Autodesk Inventor part; units mm, degrees
ref_plane "YZ Plane" through (0, 0, 0) normal (1, 0, 0) x (0, 1, 0)
ref_plane "XZ Plane" through (0, 0, 0) normal (0, 1, 0) x (-1, 0, 0)
ref_plane "XY Plane" through (0, 0, 0) normal (0, 0, 1) x (1, 0, 0)
sketch "Sketch1" plane through (0, 0, 0) normal (0, 1, 0) x (-1, 0, 0)
  line L0 (0, 22.5) -> (12, 22.5)
  line L1 (12, 22.5) -> (12, -22.5)
  line L2 (12, -22.5) -> (0, -22.5)
  arc A0 (0, -6.15) -> (0, 6.15) centre (0, 0) ccw
  line L3 (0, 22.5) -> (0, 6.15)
  line L4 (0, -6.15) -> (0, -22.5)
  point P0 (12, 0)
  dimension "d0" = 12
  dimension "d1" = 45
  dimension "d2" = 6.15
extrude "Extrusion1" add sketch "Sketch1" along normal blind 8
sketch "Sketch2" plane through (0, 8, 0) normal (0, 1, 0) x (1, 0, 0)
  line L0 (0, -22.5) -> (0, -6.15)
  arc A0 (0, 7.65) -> (0, -7.65) centre (0, 0) ccw
  line L1 (0, -7.65) -> (0, 7.65)
  dimension "d5" = 7.65
extrude "Extrusion2" cut sketch "Sketch2" against normal blind 3
sketch "Sketch3" plane through (0, 0, 22.5) normal (1, 0, 0) x (0, 0, -1)
  circle A0 centre (6.5, 4) radius 1.6
  circle A1 centre (38.5, 4) radius 1.6
  line L0 (16.35, 0) -> (0, 0)
  point P0 (22.5, 0)
  dimension "d8" = 3.2
  dimension "d9" = 32
  dimension "d10" = 4
  dimension "d11" = 16
extrude "Extrusion3" cut sketch "Sketch3" against normal up to next
sketch "Sketch4" plane through (0, 8, 0) normal (0, 1, 0) x (1, 0, 0)
  line L0 (-12, 22.5) -> (0, 22.5)
  line L1 (0, 22.5) -> (0, 14.5)
  line L2 (0, 14.5) -> (-12, 14.5)
  line L3 (-12, 14.5) -> (-12, 22.5)
  point P0 (0, 0)
  dimension "d14" = 8
extrude "Extrusion4" add sketch "Sketch4" along normal blind 20
sketch "Sketch5" plane through (0, 28, 0) normal (0, 1, 0) x (1, 0, 0)
  line L0 (10.0416, 49.5) -> (-12, 49.5)
  line L1 (-12, 49.5) -> (-12, 14.5)
  arc A0 (-2, 14.5) -> (15, 31.5) centre (-2, 31.5) ccw
  line L2 (-12, 14.5) -> (-2, 14.5)
  line L3 (15, 31.5) -> (15, 37.5)
  arc A1 (15, 37.5) -> (10.0416, 49.5) centre (-2, 37.5) ccw
  circle A2 centre (2, 37.5) radius 9.3
  point P0 (0, 0)
  dimension "d19" = 35
  dimension "d20" = 17
  dimension "d21" = 10
  dimension "d22" = 6
  dimension "d23" = 18.6
  dimension "d24" = 14
extrude "Extrusion5" add sketch "Sketch5" along normal blind 5
properties material "ABS Plastic"
For this review, take the finished solid that the model builds, in its own axes (mm). A direction names the side the tool comes from. Coordinates: 2 decimals unless noted, no trailing zeros. Order: outer loops, then holes, each group sorted by start corner. A loop starts at its lowest first (then second) coordinate and runs counter-clockwise, first axis right, second up. Notation, with made-up numbers: (15, 74) - (30, 74) arc R22 cw to (30, 104) - close; hole circle Ø6 at (-36.75, 11). An arc over 180 degrees is marked (long way). Use one line per item in the form item = value.
Q1. Consider section B-B (z = -16). Give the boundary of the cut face in (x, y).
Checked values:
outline = (-12, 0) - (0, 0) - (0, 2.4) - (-12, 2.4) - close; (-12, 5.6) - (0, 5.6) - (0, 28) - (4.98, 28) - (4.98, 33) - (-12, 33) - close
Q2. Consider section D-D (x = 2). Give the boundary of the cut face in (y, z).
Checked values:
outline = (28, -49.5) - (33, -49.5) - (33, -46.8) - (28, -46.8) - close; (28, -28.2) - (33, -28.2) - (33, -14.98) - (28, -14.98) - close
Q3. For P1, Ø3.5, axis at x = -9, z = -0.5, coming from the +Y side; P2, Ø12, axis at x = -0.5, y = 15, coming from the -Z side; P3, Ø13, axis at y = 11, z = -17, coming from the +X side; P4, Ø10, axis at x = 0.5, y = 5.5, coming from the +Z side, all flat-tipped, find the tip position at first contact; note any pin that passes through.
Checked values:
P1 = 8
P2 = -22.5
P3 = 0
P4 = 22.5
Q4. Draft analysis for pull direction Z (two halves, no side actions). For faces 6 (the cylindrical face through (-6.15, 2.46, 0.14)), 7 (the flat face through (-6, 4, 22.5)), 8 (the cylindrical face through (13.676, 30.465, -44.078)), state which applies: +Z half, -Z half, draft (parallel to the pull), parting line (faces both ways), or undercut.
Checked values:
face_6 = undercut
face_7 = +Z half
face_8 = -Z half
Q5. For probe 1 along X at (y, z) = (29, -37); probe 2 along Y at (x, z) = (-9, 16); probe 3 along Z at (x, y) = (2, 30.7), list the stretches that pass through material, from the lowest coordinate up. Write a range as from..to.
Checked values:
probe_1 = -12..-7.29, 11.29..15
probe_2 = 0..2.4, 5.6..8
probe_3 = -49.5..-46.8, -28.2..-14.98
Q6. For faces 1 (the cylindrical face through (-7.65, 6.52, -0.17)), 2 (the flat face through (-6, 14, -22.5)), 3 (the flat face through (-7, 8, 4)), 4 (the cylindrical face through (-5.92, 4.07, -14.4)), 5 (the flat face through (0, 11, -16)), list the 3-axis set-ups (+Z, -Z, +X, -X, +Y, -Y) from which the entire face can be reached by the end or side of a thin tool; tool diameter is ignored.
Checked values:
face_1 = +X, +Y
face_2 = -Z, +X, -X, -Y
face_3 = +Z, +X, -X, +Y
face_4 = +X, -X
face_5 = +Z, -Z, +X, -Y
Q7. Consider section A-A (y = 4). Give the boundary of the cut face in (x, z), then the cut area to 3 significant figures.
Checked values:
outline = (-12, -22.5) - (0, -22.5) - (0, -17.6) - (-12, -17.6) - close; (-12, -14.4) - (0, -14.4) - (0, -6.15) arc R6.15 cw to (0, 6.15) - (0, 14.4) - (-12, 14.4) - close; (-12, 17.6) - (0, 17.6) - (0, 22.5) - (-12, 22.5) - close
area = 404 mm2
Q8. Consider section C-C (x = -3.5). Give the boundary of the cut face in (y, z), then the cut area to 3 significant figures.
Checked values:
outline = (0, -22.5) - (28, -22.5) - (28, -30) - (33, -30) - (33, -14.5) - (8, -14.5) - (8, -6.8) - (5, -6.8) - (5, -5.06) - (0, -5.06) - close; (0, 5.06) - (5, 5.06) - (5, 6.8) - (8, 6.8) - (8, 22.5) - (0, 22.5) - close; (28, -49.5) - (33, -49.5) - (33, -45) - (28, -45) - close; hole circle Ø3.2 at (4, -16); hole circle Ø3.2 at (4, 16)
area = 513 mm2
